Answer from the drawing. Dimensions are ordinates in mm from the lowest x, y and z of the part. Coordinates: 2 decimals unless noted, no trailing zeros. Loops run counter-clockwise (first coordinate to the right, second up) from the corner with the lowest first, then second, coordinate; pieces in that order, holes last.
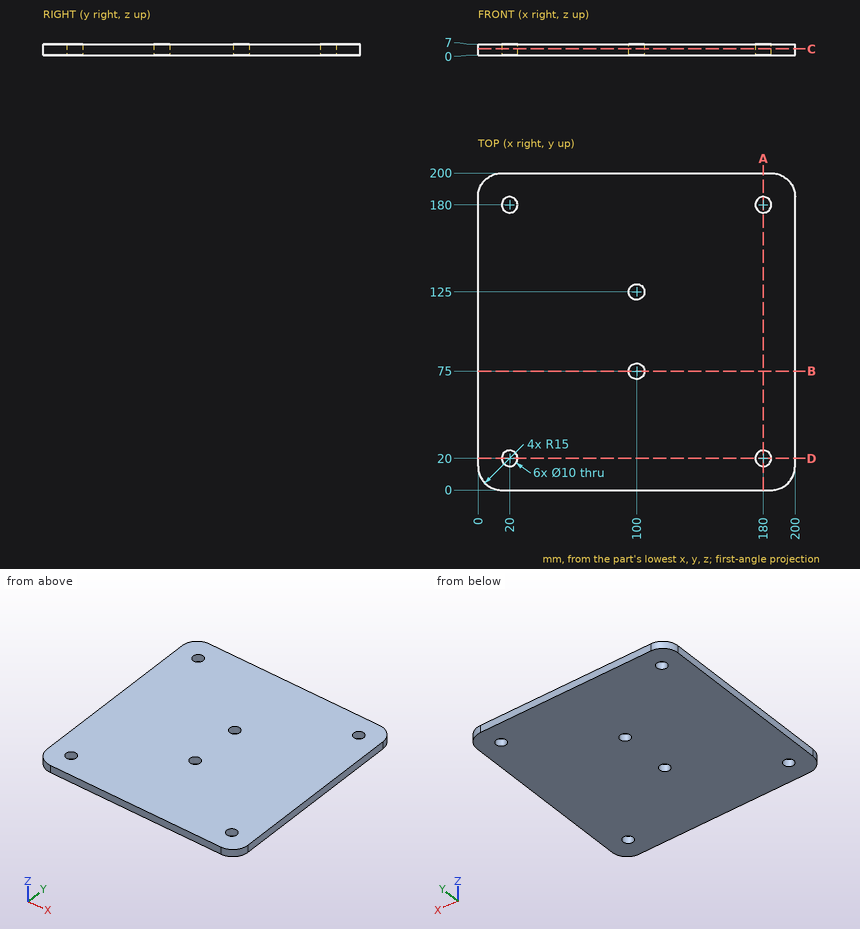
Item 1: A cutting plane is placed at B-B on y = 75. Determine the outline of the cut face in (x, z), then the cut area to 3 significant figures.
Numbers:
outline: (0, 0) - (95, 0) - (95, 7) - (0, 7) - close; (105, 0) - (200, 0) - (200, 7) - (105, 7) - close
area: 1,330 mm2
Item 2: A cutting plane is placed at A-A on x = 180. Determine the outline of the cut face in (y, z), then the cut area to 3 significant figures.
Numbers:
outline: (0, 0) - (15, 0) - (15, 7) - (0, 7) - close; (25, 0) - (175, 0) - (175, 7) - (25, 7) - close; (185, 0) - (200, 0) - (200, 7) - (185, 7) - close
area: 1,260 mm2
Item 3: A cutting plane is placed at C-C on z = 4. Determine the outline of the cut face in (x, y), then the cut area to 3 significant figures.
Numbers:
outline: (0, 15) arc R15 ccw to (15, 0) - (185, 0) arc R15 ccw to (200, 15) - (200, 185) arc R15 ccw to (185, 200) - (15, 200) arc R15 ccw to (0, 185) - close; hole circle Ø10 at (20, 20); hole circle Ø10 at (20, 180); hole circle Ø10 at (100, 75); hole circle Ø10 at (100, 125); hole circle Ø10 at (180, 20); hole circle Ø10 at (180, 180)
area: 39,300 mm2
Item 4: Find the intervals of material crossed by line 1 along Y through (x, z) = (20, 2.25); line 2 along Y through (x, z) = (100, 5.75), in increasing order.
Numbers:
line 1: y = 0 to 15, 25 to 175, 185 to 200
line 2: y = 0 to 70, 80 to 120, 130 to 200
